For this review, take the finished solid that the model builds, in its own axes (mm). A direction names the side the tool comes from. Coordinates: 2 decimals unless noted, no trailing zeros. Loops run counter-clockwise (first coordinate to the right, second up) from the corner with the lowest first, then second, coordinate; pieces in that order, holes last.
1. To check wall thickness, follow probe 1 along Z at (x, y) = (0, -6.25); probe 2 along X at (y, z) = (-6, 4); probe 3 along X at (y, z) = (-13.25, 9). State the ranges of each line that lie inside material, in increasing order.
2. Take a section at A-A, the plane z = -9.5. State the section outline as (x, y) points, then the cut area to 3 significant figures.
3. Take a section at D-D, the plane x = -8.5. State the section outline as (y, z) points, then the cut area to 3 significant figures.
4. Clearance check with flat-ended pins moving along their axes: P1, Ø5, axis at x = 83, y = -21.5, coming from the +Z side; P2, Ø3, axis at x = 137, y = -9.5, coming from the +Z side; P3, Ø2, axis at x = 17.5, y = -17.5, coming from the +Z side; P4, Ø23, axis at x = 0, z = 0, coming from the +Y side. State where each tip first meets the part, or that it passes through.
5. Mouldability with a two-part tool opening along Z and no side actions: class faces 4 (the face through (-2.75, -12.52, -12.4)), 5 (the face through (-15.275, -12.522, 16.318)), 6 (the face through (141.872, -13, -5)) as pulls with the +Z half, pulls with the -Z half, needs draft (parallel to the pull), parting line crosses it, or undercut.
6. Take a section at B-B, the plane y = -20. State the section outline as (x, z) points.
7. Machinability: for faces 1 (the face through (137, -13, 13.181)), 2 (the face through (127, -12.5, 3.9)), 3 (the face through (59, 0, -10)), which of the approach directions +Z, -Z, +X, -X, +Y, -Y give a long, thin tool a straight path to every point of the face, cutting with its end or side? Answer none if there is none.
8. Take a section at C-C, the plane z = 11. State the section outline as (x, y) points, then the cut area to 3 significant figures.
```python
from build123d import *

# Parameters (mm, degrees)
F0_R     = 12.7
F1_DEPTH = 25.4


with BuildPart() as f1:
    # F0 (on Front) → F1 (new body)
    with BuildSketch(Plane.XZ):
        Circle(F0_R)
        with BuildLine():
            ThreePointArc((0, -22.352), (15.805251, -15.805251), (22.352, 0))
            ThreePointArc((22.352, 0), (-15.805251, 15.805251), (0, -22.352))
        make_face()
        Circle(F0_R, mode=Mode.SUBTRACT)
        with BuildLine():
            Line((117.2464, 0), (22.352, 0))
            ThreePointArc((22.352, 0), (15.805251, -15.805251), (0, -22.352))
            Line((0, -22.352), (141.871706, -22.352))
            Line((141.871706, -22.352), (141.871706, 13.181371))
            Line((141.871706, 13.181371), (131.363466, 13.181371))
            ThreePointArc((131.363466, 13.181371), (126.903523, 3.807631), (117.2464, 0))
        make_face()
    extrude(amount=F1_DEPTH)


solid = f1.part
```
Results list:
1. probe 1: z = -22.35 to -12.7, 12.7 to 22.35
1. probe 2: x = -21.99 to -12.05, 12.05 to 21.99, 127.11 to 141.87
1. probe 3: x = -20.46 to -8.96, 8.96 to 20.46, 130.43 to 141.87
2. outline: (-20.23, -25.4) - (-8.43, -25.4) - (-8.43, 0) - (-20.23, 0) - close; (8.43, -25.4) - (141.87, -25.4) - (141.87, 0) - (8.43, 0) - close
2. area: 3,690 mm2
3. outline: (-25.4, -20.67) - (0, -20.67) - (0, -9.44) - (-25.4, -9.44) - close; (-25.4, 9.44) - (0, 9.44) - (0, 20.67) - (-25.4, 20.67) - close
3. area: 571 mm2
4. P1: stops at z = 0
4. P2: stops at z = 13.18
4. P3: stops at z = 15.08
4. P4: passes through
5. face 4: undercut
5. face 5: parting line crosses it
5. face 6: needs draft
6. outline: (0, -22.35) - (141.87, -22.35) - (141.87, 13.18) - (131.36, 13.18) arc R14.15 cw to (117.25, 0) - (22.35, 0) arc R22.35 ccw (long way) to start; hole circle Ø25.4 at (0, 0)
7. face 1: +Z, +X, +Y, -Y
7. face 2: +Z, +Y, -Y
7. face 3: +Z, -Z, +X, -X, +Y
8. outline: (-19.46, -25.4) - (-6.35, -25.4) - (-6.35, 0) - (-19.46, 0) - close; (6.35, -25.4) - (19.46, -25.4) - (19.46, 0) - (6.35, 0) - close; (131.04, -25.4) - (141.87, -25.4) - (141.87, 0) - (131.04, 0) - close
8. area: 941 mm2
